Can you work these out from the drawing? Everything is in mm from the part's minimum corner. Coordinates: 2 decimals unless noted, no trailing zeros. Order: outer loops, then holes, each group sorted by start corner. A loop starts at its lowest first (then second) coordinate and runs counter-clockwise, first axis right, second up. Notation, with made-up numbers: (-11, -9) - (-7, -9) arc R27 ccw to (-7, 21) - close; hole circle Ø2 at (23.25, -18). An arc over 180 degrees is marked (long way). Answer as CSV lines item,"result". Start each with the question number.
Q1. Suppose I cut it at D-D (z = 33). Please give me the cut outline in (x, y).
Q2. I need wall thicknesses on line 1 (Z direction, x = 0.65, y = 59) (1 decimal); line 2 (Y direction, x = 0.85, z = 28.5) (1 decimal); line 3 (Y direction, x = 0.95, z = 50.5) (1 decimal). Which ranges of each line are inside material? Lowest first, please.
Q3. Suppose I cut it at C-C (y = 9.5). Please give me the cut outline in (x, z).
Q4. Suppose I cut it at B-B (x = 0.9). Count the separate pieces of the cut face and the enclosed holes in it, then the cut area to 3 significant figures.
Q5. For pin 1 Ø7.5 at (y, z) = (8.509, 8.509) entering from +X; pin 2 Ø10 at (y, z) = (61.595, 49.403) entering from -X, each with a flat end and sliding along its axis, tell me the tip position at first contact or that it passes through.
Q6. Suppose I cut it at A-A (z = 27). Please give me the cut outline in (x, y).
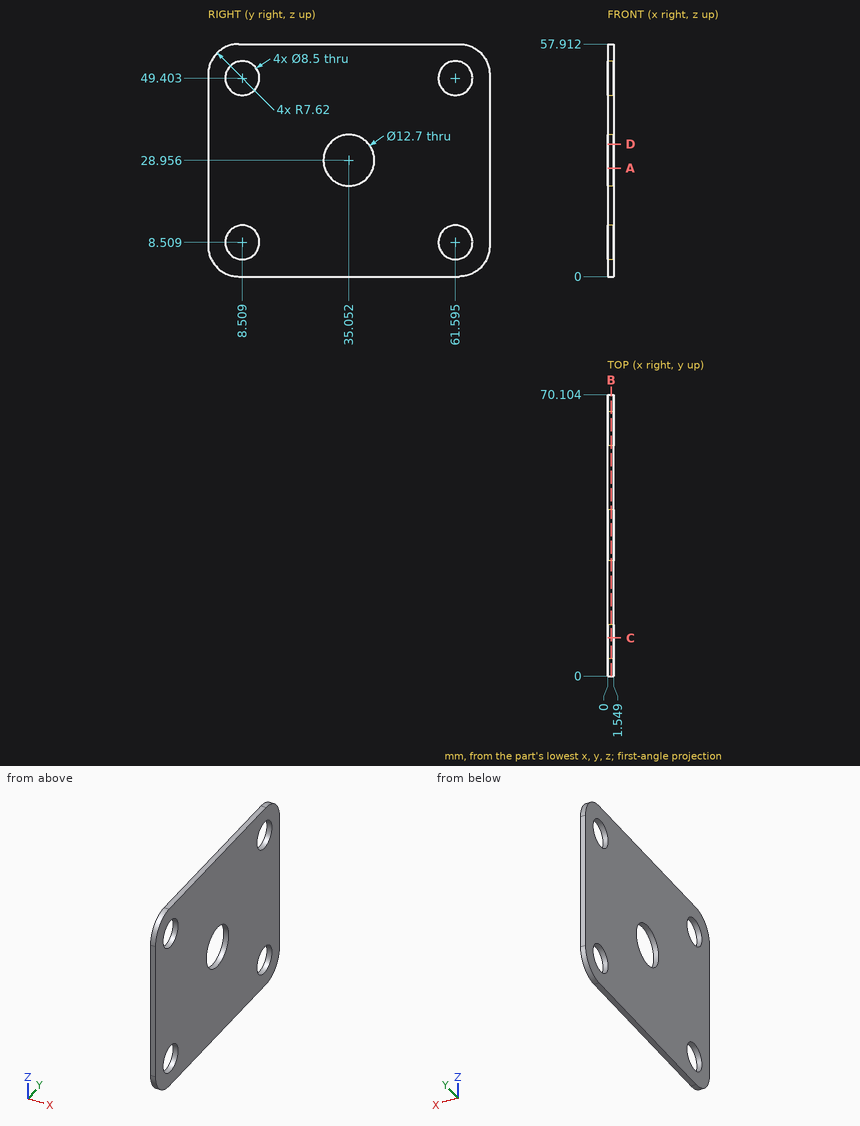
Here are the results:
1,outline,"(0, 0) - (1.55, 0) - (1.55, 30.16) - (0, 30.16) - close; (0, 39.95) - (1.55, 39.95) - (1.55, 70.1) - (0, 70.1) - close"
2,line 1,"z = 0 to 5.1, 11.9 to 46, 52.8 to 57.9"
2,line 2,"y = 0 to 28.7, 41.4 to 70.1"
2,line 3,"y = 0 to 4.4, 12.6 to 57.5, 65.7 to 70.1"
3,outline,"(0, 0) - (1.55, 0) - (1.55, 4.38) - (0, 4.38) - close; (0, 12.64) - (1.55, 12.64) - (1.55, 45.27) - (0, 45.27) - close; (0, 53.54) - (1.55, 53.54) - (1.55, 57.91) - (0, 57.91) - close"
4,separate pieces,"1"
4,enclosed holes,"5"
4,area,"3,660 mm²"
5,pin 1,"passes through"
5,pin 2,"stops at x = 0"
6,outline,"(0, 0) - (1.55, 0) - (1.55, 29.01) - (0, 29.01) - close; (0, 41.09) - (1.55, 41.09) - (1.55, 70.1) - (0, 70.1) - close"
